Geometry: final body of the model. Coordinates: model frame, mm. Face numbers are marked on the shaded views. A direction names the side the tool comes from. Round coordinates to 2 decimals unless told otherwise and drop trailing zeros. Loops run counter-clockwise (first coordinate to the right, second up) from the corner with the lowest first, then second, coordinate; pieces in that order, holes last. Notation, with made-up numbers: M -15,-24 L 0,-24 A5 cw 0,-20 Z; hole C 17,-6 d8. An arc over 180 degrees is marked long. Return JSON: item names as keys, results as strings.
from build123d import *

# Parameters (mm, degrees)
SKETCH1_R        = 1.5
MAINBLOCK_DEPTH  = 7
SKETCH2_R        = 14.3
ROTORSPACE_DEPTH = 6.25
MOTORBASE_DEPTH  = 0.75
FILLET1_R        = 2
FILLET2_R        = 0.5


with BuildPart() as part:
    # Sketch1 → MainBlock (new body)
    with BuildSketch(Plane(origin=(0, 0, 0), x_dir=(1, 0, 0), z_dir=(0, 1, 0))):
        with BuildLine():
            Line((-13, -15), (13, -15))
            ThreePointArc((13, -15), (14.414213562, -14.414213562), (15, -13))
            Line((15, -13), (15, 13))
            ThreePointArc((15, 13), (14.414213562, 14.414213562), (13, 15))
            Line((13, 15), (-13, 15))
            ThreePointArc((-13, 15), (-14.414213562, 14.414213562), (-15, 13))
            Line((-15, 13), (-15, -13))
            ThreePointArc((-15, -13), (-14.414213562, -14.414213562), (-13, -15))
        make_face()
        with Locations(Location((-11.5, 13.3, 0), (0, 0, 270))):
            Circle(SKETCH1_R, mode=Mode.SUBTRACT)
        with Locations(Location((11.5, 12.5, 0), (0, 0, 270))):
            Circle(SKETCH1_R, mode=Mode.SUBTRACT)
        with Locations(Location((11.5, -12.5, 0), (0, 0, 90))):
            Circle(SKETCH1_R, mode=Mode.SUBTRACT)
    extrude(amount=MAINBLOCK_DEPTH)

    # Sketch2 → RotorSpace (cut)
    with BuildSketch(Plane(origin=(0, 7, 0), x_dir=(1, 0, 0), z_dir=(0, 1, 0))):
        with Locations(Location((0, 0, 0), (0, 0, 270))):
            Circle(SKETCH2_R)
    extrude(amount=-ROTORSPACE_DEPTH, mode=Mode.SUBTRACT)

    # Sketch3 → MotorBase (cut)
    with BuildSketch(Plane(origin=(0, 0.75, 0), x_dir=(1, 0, 0), z_dir=(0, 1, 0))):
        with BuildLine():
            ThreePointArc((0.361277738, -7.991838236), (-4.967858622, -6.27059652), (-7.862560494, -1.476530557))
            Line((-7.862560494, -1.476530557), (-10.050196981, 10.172686009))
            ThreePointArc((-10.050196981, 10.172686009), (-14.050704626, -2.658514534), (-5.639005132, -13.141218403))
            Line((-5.639005132, -13.141218403), (0.361277738, -7.991838236))
        make_face()
        with BuildLine():
            ThreePointArc((-7.101773805, 3.683043419), (-2.946566572, 7.437590029), (2.652567275, 7.547442405))
            Line((2.652567275, 7.547442405), (13.834902999, 3.617382894))
            ThreePointArc((13.834902999, 3.617382894), (4.72301119, 13.497524414), (-8.561126408, 11.454130898))
            Line((-8.561126408, 11.454130898), (-7.101773805, 3.683043419))
        make_face()
        with BuildLine():
            Line((14.20013154, 1.687087505), (6.740496067, 4.308794817))
            ThreePointArc((6.740496067, 4.308794817), (7.678670736, 2.244552457), (8, 0))
            ThreePointArc((8, 0), (7.269110872, -3.340662678), (5.209993218, -6.070911848))
            Line((5.209993218, -6.070911848), (-3.784706018, -13.790068903))
            ThreePointArc((-3.784706018, -13.790068903), (8.670891071, -11.371264135), (14.3, 0))
            ThreePointArc((14.3, 0), (14.275011051, 0.845020408), (14.20013154, 1.687087505))
        make_face()
    extrude(amount=-MOTORBASE_DEPTH, mode=Mode.SUBTRACT)

    # Fillet1
    # the kernel refuses this fillet: 2 mm, written as the material it adds along each edge
    with BuildSketch(Plane(origin=(-8.561126408, 0.75, -11.454130898), x_dir=(0.18456631960106568, 0, 0.982820061694366), z_dir=(0, -1, 0)), Plane(origin=(14.20013154, 0.75, -1.687087505), x_dir=(-0.9434303005767882, 0, -0.33157090938981826), z_dir=(0, -1, 0))) as fillet1_piece_1:
        with BuildLine():
            CenterArc((1.313556996, -2), FILLET1_R, 90, 69.537546468)
            ThreePointArc((-0.560245969, -1.300813008), (-0.296237592, -0.643466118), (0, 0))
            Line((0, 0), (1.313556996, 0))
        make_face()
    extrude(amount=0.75)
    with BuildSketch(Plane(origin=(-5.639005132, 0.75, 13.141218403), x_dir=(-0.8983104632101903, 0, -0.43936125419419186), z_dir=(0, -1, 0))) as fillet1_piece_2:
        with BuildLine():
            CenterArc((1.317285733, 1.997546064), FILLET1_R, 203.301017311, 69.537546468)
            Line((-0.519592983, 1.206422444), (0, 0))
            ThreePointArc((0, 0), (0.708164887, -0.017545642), (1.416329774, 0))
        make_face()
    extrude(amount=0.75)

    # Fillet2
    # the kernel refuses this fillet: 0.5 mm, written as the material it adds along each edge
    with BuildSketch(Plane(origin=(13.834902999, 0.75, -3.617382894), x_dir=(-0.9434303005767886, 0, -0.33157090938981726), z_dir=(0, -1, 0)), Plane(origin=(-3.784706018, 0.75, 13.790068903), x_dir=(0.7588639809758072, 0, -0.6512491523046687), z_dir=(0, -1, 0)), Plane(origin=(-10.050196981, 0.75, -10.172686009), x_dir=(0.18456631960117675, 0, 0.982820061694345), z_dir=(0, -1, 0))) as fillet2_piece_1:
        with BuildLine():
            CenterArc((0.981325327, 0.5), FILLET2_R, 141.979598277, 128.020401723)
            ThreePointArc((0.587429586, 0.807971014), (0.286657409, 0.409116528), (0, 0))
            Line((0, 0), (0.981325327, 0))
        make_face()
    extrude(amount=0.75)


solid = part.part
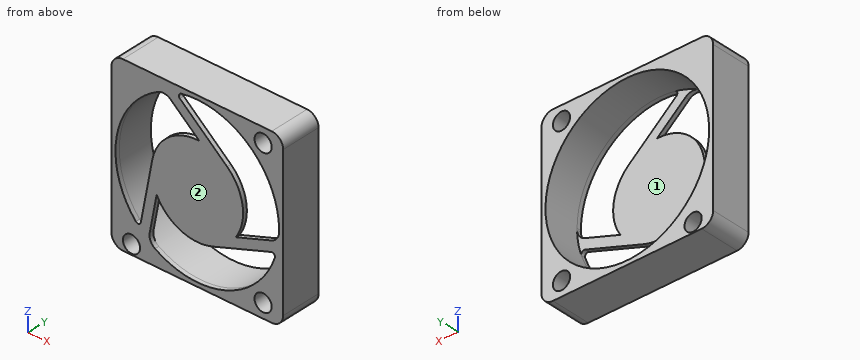
Q1. Section query C-C (x = 0). Output: boundary loops of the cut face in (y, z), plus the area to 3 significant figures.
Determined:
{"outline": "M 0,-15 L 7,-15 L 7,-14.3 L 0,-14.3 Z; M 0,-8 L 0.75,-8 L 0.75,8 L 0,8 Z; M 0,8.3 L 0.75,8.3 L 0.75,10.54 L 0,10.54 Z; M 0,14.3 L 7,14.3 L 7,15 L 0,15 Z", "area": "23.5 mm^2"}
Q2. Material intervals for L1, parallel to X at y = 5, z = 0; L2, parallel to Z at x = -12.75, y = 6.5, sorted ascending.
Determined:
{"L1": "x = -15 to -14.3, 14.3 to 15", "L2": "z = -15 to -14.13, -12.47 to -6.48, 6.48 to 15"}
Q3. Section query A-A (y = 6). Output: boundary loops of the cut face in (x, z).
Determined:
{"outline": "M -15,-13 A2 ccw -13,-15 L 13,-15 A2 ccw 15,-13 L 15,13 A2 ccw 13,15 L -13,15 A2 ccw -15,13 Z; hole C 0,0 d28.6; hole C -11.5,-13.3 d3; hole C 11.5,-12.5 d3; hole C 11.5,12.5 d3"}
Q4. Reachability of the marked faces 1 and 2 from +Z, -Z, +X, -X, +Y, -Y: full face, straight path, thin tool, end or side. Return the list, or none.
Determined:
{"face 1": "+Y", "face 2": "+Z, -Z, +X, -X, -Y"}
Q5. Section query D-D (x = -11.5). Output: boundary loops of the cut face in (y, z).
Determined:
{"outline": "M 0,-15 L 7,-15 L 7,-14.8 L 0,-14.8 Z; M 0,-11.8 L 7,-11.8 L 7,-8.5 L 0,-8.5 Z; M 0,8.5 L 7,8.5 L 7,15 L 0,15 Z"}
Q6. Pin query (flat end, axial travel): pin 1 (6 mm diameter, centred on x = -11.5, z = -6.5, fed in from +Y); pin 2 (7.5 mm diameter, centred on x = -1.5, z = 0, fed in from +Y). Return the tip coordinate at first contact, or that it passes through.
Determined:
{"pin 1": "stops at y = 7", "pin 2": "stops at y = 0.75"}
Q7. Section query B-B (z = 2.5). Output: boundary loops of the cut face in (x, y), plus the area to 3 significant figures.
Determined:
{"outline": "M -15,0 L -14.08,0 L -14.08,7 L -15,7 Z; M -7.6,0 L 7.6,0 L 7.6,0.75 L -7.6,0.75 Z; M 14.08,0 L 15,0 L 15,7 L 14.08,7 Z", "area": "24.3 mm^2"}
